Here's how the part is built. I have some questions about the finished solid (model axes, mm). A direction names the side the tool comes from. Coordinates: 2 decimals unless noted, no trailing zeros. Write each loop counter-clockwise with the first axis right and the second up, starting at its lowest first coordinate (ties: lowest second). Pieces come first, ordered by that corner, then holes.
Item 1: If we section it at B-B (z = -70): Please give me the cut outline in (x, y).
Item 2: For faces 4 (the face through (-1, 160, -100)), 5 (the face through (-70, 76, -80)), which set-ups out of +Z, -Z, +X, -X, +Y, -Y let a thin tool reach every point of the face, with its end or its side?
Item 3: If we section it at A-A (x = 70): Please give me the cut outline in (y, z).
Item 4: If we section it at D-D (x = -14.5): Please give me the cut outline in (y, z).
Item 5: I'm going to push flat-ended pins straight in: pin 1 Ø3 at (y, z) = (111, 76.5) entering from +X; pin 2 Ø6 at (y, z) = (103, 78) entering from -X; pin 3 Ø12 at (y, z) = (81, -77.5) entering from +X. Where does each tip first touch, or does it pass through?
Item 6: If we section it at C-C (y = 115): Please give me the cut outline in (x, z), then the cut area to 3 significant figures.
Item 7: If I drill on line 1 (Y direction, x = -56, z = -26); line 2 (X direction, y = 31, z = -76.5); line 3 (Z direction, x = 68, y = 105.5), over which ranges is the centre line in solid material (lowest first)?
Item 8: We'd pull the mould along Z, two halves only. Please class faces 1 (the face through (70, 76, 60)), 2 (the face through (-70, 0, 70)), 3 (the face through (-1, 160, 100)): +Z half, -Z half, draft (parallel to the pull), parting line (faces both ways), or undercut.
from build123d import *

# Parameters (mm, degrees)
SKETCH_1_W      = 200
SKETCH_1_H      = 200
EXTRUDE_1_DEPTH = 20
SKETCH_2_R      = 10
EXTRUDE_2_DEPTH = 152


with BuildPart() as part:
    # 草图1 → 凸台-拉伸1 (new body)
    with BuildSketch(Plane(origin=(0, 150, 0), x_dir=(1, 0, 0), z_dir=(0, 1, 0))):
        Rectangle(SKETCH_1_W, SKETCH_1_H)
    extrude(amount=EXTRUDE_1_DEPTH)

    # 草图2 → 凸台-拉伸2 (add)
    with BuildSketch(Plane(origin=(0, 152, 0), x_dir=(1, 0, 0), z_dir=(0, 1, 0))):
        with Locations(Location((-70, 70, 0), (0, 0, 270))):
            Circle(SKETCH_2_R)
        with Locations(Location((70, 70, 0), (0, 0, 270))):
            Circle(SKETCH_2_R)
        with Locations(Location((-70, -70, 0), (0, 0, 270))):
            Circle(SKETCH_2_R)
        with Locations(Location((70, -70, 0), (0, 0, 270))):
            Circle(SKETCH_2_R)
    extrude(amount=-EXTRUDE_2_DEPTH)


solid = part.part
Answer list:
1. outline: (-100, 150) - (-80, 150) - (-80, 0) - (-60, 0) - (-60, 150) - (60, 150) - (60, 0) - (80, 0) - (80, 150) - (100, 150) - (100, 170) - (-100, 170) - close
2. face 4: -Z, +X, -X, +Y, -Y
2. face 5: -Y
3. outline: (0, -80) - (150, -80) - (150, -100) - (170, -100) - (170, 100) - (150, 100) - (150, 80) - (0, 80) - (0, 60) - (150, 60) - (150, -60) - (0, -60) - close
4. outline: (150, -100) - (170, -100) - (170, 100) - (150, 100) - close
5. pin 1: stops at x = 78.66
5. pin 2: stops at x = -78.66
5. pin 3: stops at x = 79.89
6. outline: circle Ø20 at (-70, -70); circle Ø20 at (-70, 70); circle Ø20 at (70, -70); circle Ø20 at (70, 70)
6. area: 1,260 mm2
7. line 1: y = 150 to 170
7. line 2: x = -77.6 to -62.4, 62.4 to 77.6
7. line 3: z = -79.8 to -60.2, 60.2 to 79.8
8. face 1: undercut
8. face 2: draft
8. face 3: +Z half
